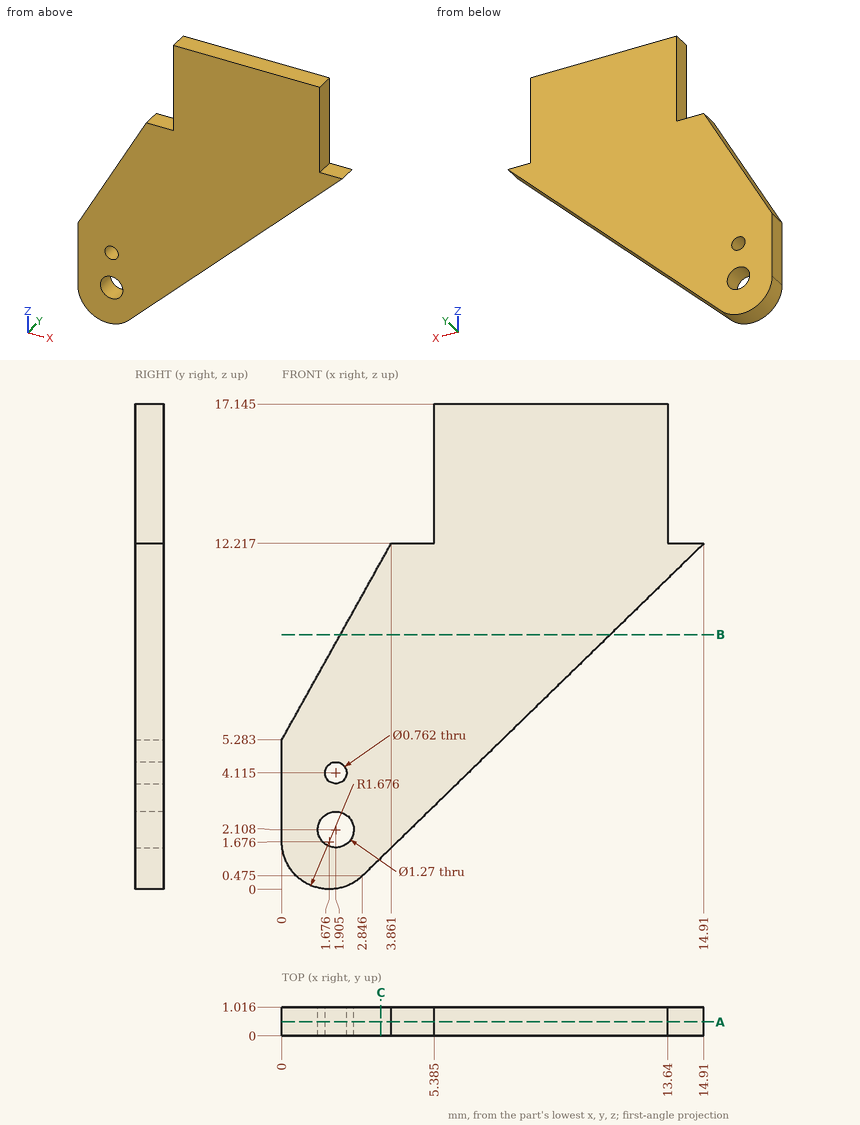
Job drawing, mm, ordinate dimensions from the low corner. One solid piece. Give positions to 0.01 mm unless a question says otherwise; leave off trailing zeros. Write each loop counter-clockwise with the first axis right and the second up, starting at its lowest first coordinate (ties: lowest second). Pieces come first, ordered by that corner, then holes. Notation, with made-up numbers: (53.5, 11.5) - (98.5, 11.5) arc R24 ccw to (98.5, 28.5) - close; hole circle Ø1 at (-19.75, -32). An arc over 180 degrees is marked (long way). Use one line per item in the form item = value. Start each with the question number.
1. Band-saw the part on A-A on y = 0.5. Write the cut outline in (x, z) (1 decimal), plus the area to 3 significant figures.
2. Band-saw the part on B-B on z = 9. Write the cut outline in (x, y) (1 decimal).
3. Probe line 1 (X direction, y = 0.9, z = 14.75) (1 decimal); line 2 (X direction, y = 0.1, z = 2.5) (1 decimal); line 3 (Z direction, x = 8.75, y = 0.85) (1 decimal). List the from-to ranges inside material, lowest first. Write a range as [from, to].
4. Band-saw the part on C-C on x = 3.5. Write the cut outline in (y, z).
Conclusion:
q1.outline = (0, 1.7) arc R1.7 ccw to (2.8, 0.5) - (14.9, 12.2) - (13.6, 12.2) - (13.6, 17.1) - (5.4, 17.1) - (5.4, 12.2) - (3.9, 12.2) - (0, 5.3) - close; hole circle Ø1.3 at (1.9, 2.1); hole circle Ø0.8 at (1.9, 4.1)
q1.area = 130 mm²
q2.outline = (2.1, 0) - (11.6, 0) - (11.6, 1) - (2.1, 1) - close
q3.line_1 = [5.4, 13.6]
q3.line_2 = [0, 1.4], [2.4, 4.9]
q3.line_3 = [6.2, 17.1]
q4.outline = (0, 1.11) - (1.02, 1.11) - (1.02, 11.57) - (0, 11.57) - close
